Input: part model. Units: mm. Frame: model coordinates. Face numbers are marked on the shaded views. Round coordinates to 2 decimals unless told otherwise and drop trailing zeros. Loops run counter-clockwise (first coordinate to the right, second up) from the corner with the lowest first, then second, coordinate; pieces in that order, holes last. Notation, with made-up numbers: (38.5, 69) -> (75.5, 69) arc R28 cw to (75.5, 104) -> close; hole circle Ø2 at (82, -3). An arc over 180 degrees is marked (long way). Answer as a JSON object with one key per item and string values. Group by question number.
Item 1: Section query A-A on y = 1.6. Return loops of the section in (x, z), and give its area (3 significant figures).
Item 2: Material intervals for line 1 (Z direction, x = 2.25, y = 1.4), sorted ascending. Write a range as [from, to].
Item 3: Draft query along X for the marked faces 1, 2 and 3. Return one class per face: released by +X, released by -X, zero draft, split by the parting line, or undercut.
Item 4: Pin query (flat end, axial travel): pin 1 (5 mm diameter, centred on x = -0.5, z = 1, fed in from -Y); pin 2 (0.9 mm diameter, centred on x = 0, y = 1, fed in from -Z). Return the tip coordinate at first contact, or that it passes through.
Item 5: Section query B-B on x = -2. Return loops of the section in (y, z), and give its area (3 significant figures).
Autodesk Inventor part; units mm, degrees
ref_plane "lens_to_bicol_led_1_XY" through (1.251, 3.9878, 4.9276) normal (0, 1, 0) x (1, 0, 0)
ref_plane "lens_to_bicol_led_1_YZ" through (1.251, 3.9878, 4.9276) normal (1, 0, 0) x (0, 0, -1)
ref_plane "lens_to_bicol_led_1_ZX" through (1.251, 3.9878, 4.9276) normal (0, 0, -1) x (0, 1, 0)
sketch "Sketch_31" plane through (0, 0, 0) normal (0, 0, 1) x (1, 0, 0)
  line L0 (-7.5057, 3.9878) -> (-7.5057, 0)
  line L1 (-7.5057, 0) -> (7.5057, 0)
  line L2 (7.5057, 0) -> (7.5057, 3.9878)
  line L3 (7.5057, 3.9878) -> (-7.5057, 3.9878)
extrude "Extrusion1" add sketch "Sketch_31" along normal mid plane 15.0114
sketch "Sketch_4" plane through (0, 0, 0) normal (0, 0, 1) x (1, 0, 0)
  line L0 (-7.5057, 1.27) -> (-7.2517, 1.27)
  line L1 (-7.2517, 1.27) -> (-7.2517, 1.8682)
  line L2 (-7.2517, 1.8682) -> (-7.5057, 1.8682)
  line L3 (-7.5057, 1.8682) -> (-7.5057, 1.27)
extrude "Extrusion2" cut sketch "Sketch_4" along normal mid plane 6.0046
sketch "Sketch_5" plane through (0, 0, 0) normal (0, 0, 1) x (1, 0, 0)
  line L0 (7.2517, 1.27) -> (7.5057, 1.27)
  line L1 (7.5057, 1.27) -> (7.5057, 1.8682)
  line L2 (7.5057, 1.8682) -> (7.2517, 1.8682)
  line L3 (7.2517, 1.8682) -> (7.2517, 1.27)
extrude "Extrusion3" cut sketch "Sketch_5" along normal mid plane 6.0046
sketch "Sketch_14" plane through (0, 0, 0) normal (1, 0, 0) x (0, 1, 0)
  line L0 (0, 7.5057) -> (0, 7.2517)
  line L1 (0, 7.2517) -> (1.8682, 7.2517)
  line L2 (1.8682, 7.2517) -> (1.8682, 7.5057)
  line L3 (1.8682, 7.5057) -> (0, 7.5057)
extrude "Extrusion4" cut sketch "Sketch_14" along normal mid plane 6.0046
sketch "Sketch_15" plane through (0, 0, 0) normal (1, 0, 0) x (0, 1, 0)
  line L0 (0, -7.2517) -> (0, -7.5057)
  line L1 (0, -7.5057) -> (1.8682, -7.5057)
  line L2 (1.8682, -7.5057) -> (1.8682, -7.2517)
  line L3 (1.8682, -7.2517) -> (0, -7.2517)
extrude "Extrusion5" cut sketch "Sketch_15" along normal mid plane 6.0046
sketch "Sketch_8" plane through (0, 0, 0) normal (0, 1, 0) x (-1, 0, 0)
  line L0 (8.2563, 8.2563) -> (-8.2563, 8.2563)
  line L1 (-8.2563, 8.2563) -> (-8.2563, -8.2563)
  line L2 (-8.2563, -8.2563) -> (8.2563, -8.2563)
  line L3 (8.2563, -8.2563) -> (8.2563, 8.2563)
  line L4 (7.5057, -7.2517) -> (7.5057, 7.2517)
  arc A0 (7.5057, 7.2517) -> (7.2517, 7.5057) centre (7.2517, 7.2517) ccw
  line L5 (7.2517, 7.5057) -> (-7.2517, 7.5057)
  arc A1 (-7.2517, 7.5057) -> (-7.5057, 7.2517) centre (-7.2517, 7.2517) ccw
  line L6 (-7.5057, 7.2517) -> (-7.5057, -7.2517)
  arc A2 (-7.5057, -7.2517) -> (-7.2517, -7.5057) centre (-7.2517, -7.2517) ccw
  line L7 (-7.2517, -7.5057) -> (7.2517, -7.5057)
  arc A3 (7.2517, -7.5057) -> (7.5057, -7.2517) centre (7.2517, -7.2517) ccw
extrude "Extrusion6" cut sketch "Sketch_8" along normal mid plane 10.5156
ref_plane "lens_to_bicol_led_1_XY" through (1.251, 3.9878, 4.9276) normal (0, 1, 0) x (1, 0, 0)
ref_plane "lens_to_bicol_led_1_YZ" through (1.251, 3.9878, 4.9276) normal (1, 0, 0) x (0, 0, -1)
ref_plane "lens_to_bicol_led_1_ZX" through (1.251, 3.9878, 4.9276) normal (0, 0, -1) x (0, 1, 0)
ref_plane "lens_to_bicol_led_2_XY" through (-1.251, 3.9878, 4.9276) normal (0, 1, 0) x (1, 0, 0)
ref_plane "lens_to_bicol_led_2_YZ" through (-1.251, 3.9878, 4.9276) normal (1, 0, 0) x (0, 0, -1)
ref_plane "lens_to_bicol_led_2_ZX" through (-1.251, 3.9878, 4.9276) normal (0, 0, -1) x (0, 1, 0)
ref_plane "lens_to_insert_XY" through (0, 2.9718, 0) normal (0, 1, 0) x (1, 0, 0)
ref_plane "lens_to_insert_YZ" through (0, 2.9718, 0) normal (1, 0, 0) x (0, 0, -1)
ref_plane "lens_to_insert_ZX" through (0, 2.9718, 0) normal (0, 0, -1) x (0, 1, 0)
ref_plane "lens_to_led_XY" through (0, 3.9878, 4.9276) normal (0, 1, 0) x (1, 0, 0)
ref_plane "lens_to_led_YZ" through (0, 3.9878, 4.9276) normal (1, 0, 0) x (0, 0, -1)
ref_plane "lens_to_led_ZX" through (0, 3.9878, 4.9276) normal (0, 0, -1) x (0, 1, 0)
ref_plane "lens_to_body_XY" through (0, 0, 0) normal (0, 1, 0) x (1, 0, 0)
ref_plane "lens_to_body_YZ" through (0, 0, 0) normal (1, 0, 0) x (0, 0, -1)
ref_plane "lens_to_body_ZX" through (0, 0, 0) normal (0, 0, -1) x (0, 1, 0)
properties part number "YB16SKW01-05-BB-BBni_lens"
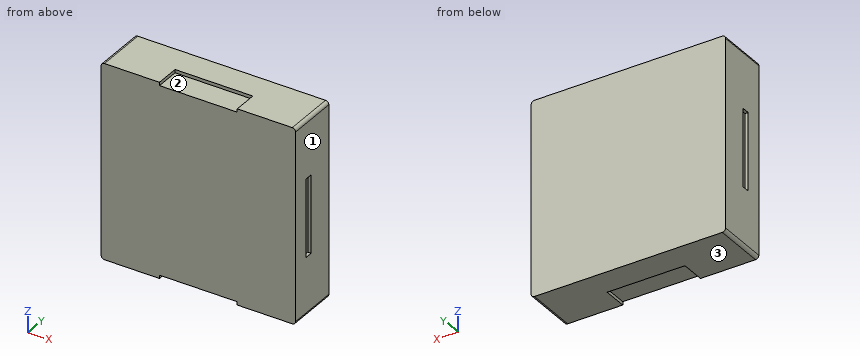
Solved:
{
 "1": {"outline": "(-7.51, -7.25) arc R0.25 ccw to (-7.25, -7.51) -> (-3, -7.51) -> (-3, -7.25) -> (3, -7.25) -> (3, -7.51) -> (7.25, -7.51) arc R0.25 ccw to (7.51, -7.25) -> (7.51, -3) -> (7.25, -3) -> (7.25, 3) -> (7.51, 3) -> (7.51, 7.25) arc R0.25 ccw to (7.25, 7.51) -> (3, 7.51) -> (3, 7.25) -> (-3, 7.25) -> (-3, 7.51) -> (-7.25, 7.51) arc R0.25 ccw to (-7.51, 7.25) -> (-7.51, 3) -> (-7.25, 3) -> (-7.25, -3) -> (-7.51, -3) -> close", "area": "219 mm²"},
 "2": {"line 1": "[-7.25, 7.25]"},
 "3": {"face 1": "released by +X", "face 2": "undercut", "face 3": "zero draft"},
 "4": {"pin 1": "y = 0", "pin 2": "z = -7.25"},
 "5": {"outline": "(0, -7.25) -> (1.87, -7.25) -> (1.87, -7.51) -> (3.99, -7.51) -> (3.99, 7.51) -> (1.87, 7.51) -> (1.87, 7.25) -> (0, 7.25) -> close", "area": "58.9 mm²"}
}
